Geometry: see drawing. Coordinates: mm, zero at the bounding-box minimum. Give positions to 0.01 mm unless a question says otherwise; leave off trailing zeros. Loops run counter-clockwise (first coordinate to the right, second up) from the corner with the lowest first, then second, coordinate; pieces in that order, holes last. Notation, with made-up numbers: M 28,73 L 36,73 A31 ccw 36,109 Z; hole C 11.5,42 d5. An arc over 180 degrees is marked long. Put each result on its own line as item: value.
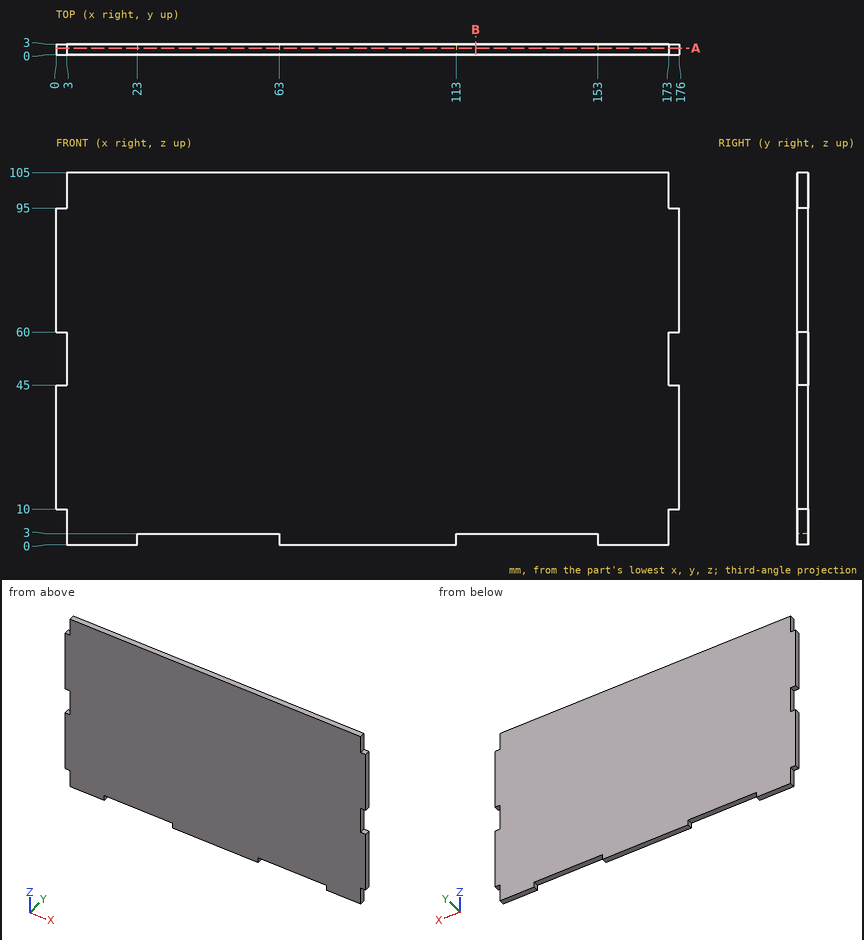
Item 1: Line query: probe 1 along Z at (x, y) = (37, 1.1); probe 2 along X at (y, z) = (2.3, 6.5). Output: solid intervals per line, ascending. Write a range as [from, to].
Output values:
probe 1: [3, 105]
probe 2: [3, 173]
Item 2: Pin query (flat end, axial travel): pin 1 Ø1.5 at (y, z) = (1.5, 1.5) entering from -X; pin 2 Ø0.9 at (x, y) = (133.5, 1) entering from -Z; pin 3 Ø1.5 at (x, y) = (1, 1) entering from -Z. Return the tip coordinate at first contact, or that it passes through.
Output values:
pin 1: x = 3
pin 2: z = 3
pin 3: z = 10
Item 3: Section B-B on x = 118.5. Output: boundary loops of the cut face in (y, z).
Output values:
outline: M 0,3 L 3,3 L 3,105 L 0,105 Z
Item 4: Section A-A on y = 1.85. Output: boundary loops of the cut face in (x, z).
Output values:
outline: M 0,10 L 3,10 L 3,0 L 23,0 L 23,3 L 63,3 L 63,0 L 113,0 L 113,3 L 153,3 L 153,0 L 173,0 L 173,10 L 176,10 L 176,45 L 173,45 L 173,60 L 176,60 L 176,95 L 173,95 L 173,105 L 3,105 L 3,95 L 0,95 L 0,60 L 3,60 L 3,45 L 0,45 Z
